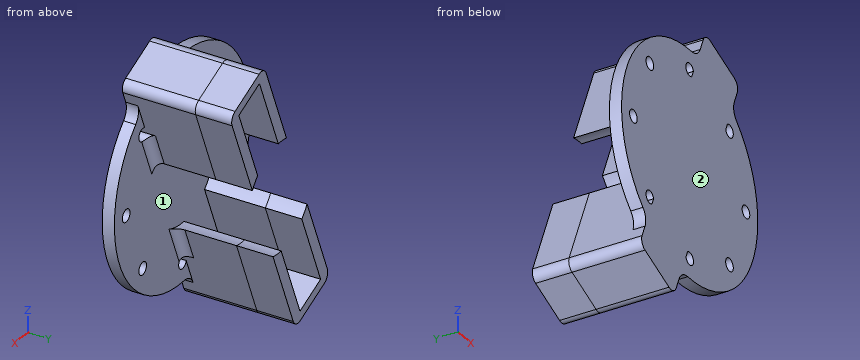
from build123d import *

# Parameters (mm, degrees)
CROQUIS2_R                   = 37.5
SALIENTE_EXTRUIR1_DEPTH      = 4
CROQUIS3_R                   = 2.1
CORTAR_EXTRUIR1_DEPTH        = 4
SALIENTE_EXTRUIR2_DEPTH      = 20
SALIENTE_EXTRUIR2_DEPTH_BACK = 4
SALIENTE_EXTRUIR3_DEPTH      = 20
SALIENTE_EXTRUIR3_DEPTH_BACK = 4
CORTAR_EXTRUIR2_DEPTH        = 20
CROQUIS9_R                   = 18
CORTAR_EXTRUIR3_DEPTH        = 20
REDONDEO1_R                  = 3
REDONDEO2_R                  = 3
REDONDEO3_R                  = 5
CORTAR_EXTRUIR4_DEPTH        = 20
SALIENTE_EXTRUIR4_START      = 12
SALIENTE_EXTRUIR4_DEPTH      = 12


with BuildPart() as part:
    # Croquis2 → Saliente-Extruir1 (new body)
    with BuildSketch(Plane(origin=(0, 0, 0), x_dir=(1, 0, 0), z_dir=(0, 1, 0))):
        with Locations(Location((0, 0, 0), (0, 0, 270))):
            Circle(CROQUIS2_R)
    extrude(amount=SALIENTE_EXTRUIR1_DEPTH)

    # Croquis3 → Cortar-Extruir1 (cut)
    with BuildSketch(Plane(origin=(0, 4, 0), x_dir=(1, 0, 0), z_dir=(0, 1, 0))):
        with Locations(Location((0, 31, 0), (0, 0, 270))):
            Circle(CROQUIS3_R)
        with Locations(Location((21.920310217, 21.920310217, 0), (0, 0, 270))):
            Circle(CROQUIS3_R)
        with Locations(Location((31, 0, 0), (0, 0, 270))):
            Circle(CROQUIS3_R)
        with Locations(Location((21.920310217, -21.920310217, 0), (0, 0, 270))):
            Circle(CROQUIS3_R)
        with Locations(Location((0, -31, 0), (0, 0, 270))):
            Circle(CROQUIS3_R)
        with Locations(Location((-21.920310217, -21.920310217, 0), (0, 0, 270))):
            Circle(CROQUIS3_R)
        with Locations(Location((-31, 0, 0), (0, 0, 270))):
            Circle(CROQUIS3_R)
        with Locations(Location((-21.920310217, 21.920310217, 0), (0, 0, 270))):
            Circle(CROQUIS3_R)
    extrude(amount=-CORTAR_EXTRUIR1_DEPTH, mode=Mode.SUBTRACT)

    # Croquis4 → Saliente-Extruir2 (add, two sides: drawn at the far end of the back side and taken through both)
    with BuildSketch(Plane(origin=(0, 4, 0), x_dir=(1, 0, 0), z_dir=(0, 1, 0)).offset(-SALIENTE_EXTRUIR2_DEPTH_BACK)):
        with BuildLine():
            ThreePointArc((8.474466938, -36.529897483), (11.451375588, -35.708766391), (14.350628714, -34.645482469))
            Line((14.350628714, -34.645482469), (-14.350628714, 34.645482469))
            ThreePointArc((-14.350628714, 34.645482469), (-17.15256553, 33.347256195), (-19.838185188, 31.822891265))
            Line((-19.838185188, 31.822891265), (8.474466938, -36.529897483))
        make_face()
        with BuildLine():
            Line((-14.350628714, 34.645482469), (14.350628714, -34.645482469))
            ThreePointArc((14.350628714, -34.645482469), (17.15256553, -33.347256195), (19.838185188, -31.822891265))
            Line((19.838185188, -31.822891265), (-8.474466938, 36.529897483))
            ThreePointArc((-8.474466938, 36.529897483), (-11.451375588, 35.708766391), (-14.350628714, 34.645482469))
        make_face()
        with BuildLine():
            Line((10.773528467, -42.080323007), (16.455387592, -39.726819898))
            Line((16.455387592, -39.726819898), (14.350628714, -34.645482469))
            ThreePointArc((14.350628714, -34.645482469), (11.451375588, -35.708766391), (8.474466938, -36.529897483))
            Line((8.474466938, -36.529897483), (10.773528467, -42.080323007))
        make_face()
        with BuildLine():
            Line((14.350628714, -34.645482469), (16.455387592, -39.726819898))
            Line((16.455387592, -39.726819898), (22.137246717, -37.373316789))
            Line((22.137246717, -37.373316789), (19.838185188, -31.822891265))
            ThreePointArc((19.838185188, -31.822891265), (17.15256553, -33.347256195), (14.350628714, -34.645482469))
        make_face()
        with BuildLine():
            ThreePointArc((-19.838185188, 31.822891265), (-17.15256553, 33.347256195), (-14.350628714, 34.645482469))
            Line((-14.350628714, 34.645482469), (-16.455387592, 39.726819898))
            Line((-16.455387592, 39.726819898), (-22.137246717, 37.373316789))
            Line((-22.137246717, 37.373316789), (-19.838185188, 31.822891265))
        make_face()
        with BuildLine():
            Line((-16.455387592, 39.726819898), (-14.350628714, 34.645482469))
            ThreePointArc((-14.350628714, 34.645482469), (-11.451375588, 35.708766391), (-8.474466938, 36.529897483))
            Line((-8.474466938, 36.529897483), (-10.773528467, 42.080323007))
            Line((-10.773528467, 42.080323007), (-16.455387592, 39.726819898))
        make_face()
    extrude(amount=SALIENTE_EXTRUIR2_DEPTH + SALIENTE_EXTRUIR2_DEPTH_BACK)

    # Croquis6 → Saliente-Extruir3 (add, two sides: drawn at the far end of the back side and taken through both)
    with BuildSketch(Plane(origin=(0, 4, 0), x_dir=(1, 0, 0), z_dir=(0, 1, 0)).offset(-SALIENTE_EXTRUIR3_DEPTH_BACK)):
        Polygon((-27.363498576, 39.53810119), (8.608744066, -47.306574867), (27.363498576, -39.53810119), (-8.608744066, 47.306574867), align=None)
        Polygon((-22.137246717, 37.373316789), (10.773528467, -42.080323007), (22.137246717, -37.373316789), (-10.773528467, 42.080323007), align=None, mode=Mode.SUBTRACT)
    extrude(amount=SALIENTE_EXTRUIR3_DEPTH + SALIENTE_EXTRUIR3_DEPTH_BACK)

    # Croquis8 → Cortar-Extruir2 (cut)
    with BuildSketch(Plane(origin=(0, 24, 0), x_dir=(1, 0, 0), z_dir=(0, 1, 0))):
        Polygon((-10.773528467, 42.080323007), (-22.137246717, 37.373316789), (10.773528467, -42.080323007), (22.137246717, -37.373316789), align=None)
    extrude(amount=-CORTAR_EXTRUIR2_DEPTH, mode=Mode.SUBTRACT)

    # Croquis9 → Cortar-Extruir3 (cut)
    with BuildSketch(Plane(origin=(0, 24, 0), x_dir=(1, 0, 0), z_dir=(0, 1, 0))):
        Circle(CROQUIS9_R)
    extrude(amount=-CORTAR_EXTRUIR3_DEPTH, mode=Mode.SUBTRACT)

    # Redondeo1
    redondeo1_edges = [part.edges().sort_by_distance(p)[0] for p in [
        (1.285328501, 4, -23.420170689),
        (-1.285328501, 4, 23.420170689),
        (-17.469426009, 4, -15.651697012),
        (17.469426009, 4, 15.651697012),
    ]]
    fillet(redondeo1_edges, radius=REDONDEO1_R)

    # Redondeo2
    redondeo2_edges = [part.edges().sort_by_distance(p)[0] for p in [
        (8.608744066, 12, 47.306574867),
        (-8.608744066, 12, -47.306574867),
        (-27.363498576, 12, -39.53810119),
        (27.363498576, 12, 39.53810119),
    ]]
    fillet(redondeo2_edges, radius=REDONDEO2_R)

    # Redondeo3
    redondeo3_edges = [part.edges().sort_by_distance(p)[0] for p in [
        (-23.192341919, 2, -29.468038216),
        (4.437587409, 2, 37.236511893),
        (23.192341919, 2, 29.468038216),
        (-4.437587409, 2, -37.236511893),
    ]]
    fillet(redondeo3_edges, radius=REDONDEO3_R)

    # Croquis10 → Cortar-Extruir4 (cut)
    with BuildSketch(Plane(origin=(0, 24, 0), x_dir=(1, 0, 0), z_dir=(0, 1, 0))):
        Polygon((10.773528467, -42.080323007), (22.137246717, -37.373316789), (22.519930149, -38.297196321), (11.156211899, -43.00420254), align=None)
        Polygon((-10.773528467, 42.080323007), (-22.137246717, 37.373316789), (-22.519930149, 38.297196321), (-11.156211899, 43.00420254), align=None)
    extrude(amount=-CORTAR_EXTRUIR4_DEPTH, mode=Mode.SUBTRACT)

    # Croquis11 → Saliente-Extruir4 (add)
    with BuildSketch(Plane(origin=(0, 24, 0), x_dir=(1, 0, 0), z_dir=(0, 1, 0)).offset(SALIENTE_EXTRUIR4_START)):
        with BuildLine():
            Line((22.519930149, -38.297196321), (11.156211899, -43.00420254))
            Line((11.156211899, -43.00420254), (0.791912926, -17.982571393))
            ThreePointArc((0.791912926, -17.982571393), (-1.459803938, -17.940707134), (-3.688668647, -17.617994313))
            Line((-3.688668647, -17.617994313), (7.460693769, -44.534936269))
            ThreePointArc((7.460693769, -44.534936269), (9.08428207, -46.158524569), (11.380382664, -46.158524569))
            Line((11.380382664, -46.158524569), (24.591859979, -40.686151487))
            ThreePointArc((24.591859979, -40.686151487), (26.215448279, -39.062563186), (26.215448279, -36.766462592))
            Line((26.215448279, -36.766462592), (15.066085863, -9.849520636))
            ThreePointArc((15.066085863, -9.849520636), (13.718232938, -11.65375841), (12.155631176, -13.275565175))
            Line((12.155631176, -13.275565175), (22.519930149, -38.297196321))
        make_face()
        with BuildLine():
            Line((-22.519930149, 38.297196321), (-11.156211899, 43.00420254))
            Line((-11.156211899, 43.00420254), (-0.791912926, 17.982571393))
            ThreePointArc((-0.791912926, 17.982571393), (1.459803938, 17.940707134), (3.688668647, 17.617994313))
            Line((3.688668647, 17.617994313), (-7.460693769, 44.534936269))
            ThreePointArc((-7.460693769, 44.534936269), (-9.08428207, 46.158524569), (-11.380382664, 46.158524569))
            Line((-11.380382664, 46.158524569), (-24.591859979, 40.686151487))
            ThreePointArc((-24.591859979, 40.686151487), (-26.215448279, 39.062563186), (-26.215448279, 36.766462592))
            Line((-26.215448279, 36.766462592), (-15.066085863, 9.849520636))
            ThreePointArc((-15.066085863, 9.849520636), (-13.718232938, 11.65375841), (-12.155631176, 13.275565175))
            Line((-12.155631176, 13.275565175), (-22.519930149, 38.297196321))
        make_face()
    extrude(amount=-SALIENTE_EXTRUIR4_DEPTH)


solid = part.part
Work out the finished part from the listing and answer in its coordinate system (mm). Face numbers are marked on the shaded views. Coordinates: 2 decimals unless noted, no trailing zeros. Loops run counter-clockwise (first coordinate to the right, second up) from the corner with the lowest first, then second, coordinate; pieces in that order, holes last. Notation, with made-up numbers: M 31.5,52 L 66.5,52 A24 cw 66.5,72 Z; hole C 16.5,1.5 d2. An arc over 180 degrees is marked long. Answer in a Markdown table with one row per item. Add a question column.
1. The mould has two halves that part along X. Classify the marked faces 1 and 2: pulls with the +X half, pulls with the -X half, needs draft (parallel to the pull), parting line crosses it, or undercut.
2. Find section B-B, the plane y = 25.5. Write down the section's boundary in (x, z).
3. Find section D-D, the plane y = 3. State how many separate pieces and enclosed holes the cut face has, then the cut area to 3 significant figures.
4. Find section A-A, the plane z = 0. Write down the section's boundary in (x, y).
5. Find section C-C, the plane x = -31. Write down the section's boundary in (y, z).
6. Consider L1, parallel to X at y = 2, z = 0; L2, parallel to Z at x = 1, y = 3; L3, parallel to Z at x = 0.5, y = 18.5. Determine where each line is inside the solid, lowest interval first.
7. Flat-ended cylindrical pins translate along their axes: P1, Ø1, axis at y = 27, z = -26, coming from the +X side; P2, Ø5, axis at x = 21.92, z = -21.92, coming from the +Y side; P3, Ø2, axis at x = -14.5, y = 23, coming from the +Z side. Find the tip coordinate at first contact, or state that the pin passes through.
Reported:
| question | item | result |
|---|---|---|
| 1 | face 1 | undercut |
| 1 | face 2 | needs draft |
| 2 | outline | M -26.22,-36.77 A3 ccw -24.59,-40.69 L -11.38,-46.16 A3 ccw -7.46,-44.53 L 3.69,-17.62 A18 cw -0.79,-17.98 L -11.16,-43 L -22.52,-38.3 L -12.16,-13.28 A18 cw -15.07,-9.85 Z; M -3.69,17.62 A18 cw 0.79,17.98 L 11.16,43 L 22.52,38.3 L 12.16,13.28 A18 cw 15.07,9.85 L 26.22,36.77 A3 ccw 24.59,40.69 L 11.38,46.16 A3 ccw 7.46,44.53 Z |
| 3 | separate pieces | 1 |
| 3 | enclosed holes | 8 |
| 3 | area | 4,720 mm^2 |
| 4 | outline | M -37.5,0 L -33.1,0 L -33.1,4 L -37.5,4 Z; M -28.9,0 L 28.9,0 L 28.9,4 L -28.9,4 Z; M 33.1,0 L 37.5,0 L 37.5,4 L 33.1,4 Z |
| 5 | outline | M 0,-21.1 L 4,-21.1 L 4,-2.1 L 0,-2.1 Z; M 0,2.1 L 4,2.1 L 4,21.1 L 0,21.1 Z |
| 6 | L1 | x = -37.5 to -33.1, -28.9 to 28.9, 33.1 to 37.5 |
| 6 | L2 | z = -37.49 to -32.85, -29.15 to 29.15, 32.85 to 37.49 |
| 6 | L3 | z = -25.32 to -17.99, 17.99 to 27.73 |
| 7 | P1 | stops at x = 0.42 |
| 7 | P2 | stops at y = 4 |
| 7 | P3 | stops at z = -9.85 |
